Read the model definition and answer for the solid it produces. Units are mm, in the model's axes. Coordinates: 2 decimals unless noted, no trailing zeros. Loops run counter-clockwise (first coordinate to the right, second up) from the corner with the lowest first, then second, coordinate; pieces in that order, holes last. Notation, with made-up numbers: (-22, -38) - (-3, -38) arc R22 ccw to (-3, 0) - close; hole circle Ø8 at (62.25, 48.5). An arc over 180 degrees is marked (long way). One line per item, written item: value. Start each with the question number.
Autodesk Inventor part; units mm, degrees
ref_plane "Start plane" through (0, 0, 13.6102) normal (0, 0, 1) x (1, 0, 0)
ref_plane "End plane" through (0, 0, 536.3898) normal (0, 0, 1) x (1, 0, 0)
ref_plane "Work Plane4" through (0.6642, 2.6747, 533.4641) normal (-0.0396, -0.1596, 0.9864) x (0.9992, -0.0032, 0.0396)
ref_plane "Start plane" through (0, 0, 13.6102) normal (0, 0, 1) x (1, 0, 0)
ref_plane "End plane" through (0, 0, 536.3898) normal (0, 0, 1) x (1, 0, 0)
sketch "Sketch" plane through (0, 0, 0) normal (0, 0, 1) x (1, 0, 0)
  circle A0 centre (0, 0) radius 13.3858
  circle A1 centre (0, 0) radius 16.764
  dimension "d0" = 33.528
  dimension "d1" = 3.3782
extrude "Body" add sketch "Sketch" along normal up to surface (522.7796 mm away) from surface at 13.6102
sketch "Sketch3" plane through (0, 0, 0) normal (0, 0, 1) x (1, 0, 0)
  line L0 (0, 0) -> (10, 0)
ref_plane "Work Plane3" through (0, 0, 0) normal (0, -1, 0) x (1, 0, 0)
ref_plane "Work Plane4" through (0.6642, 2.6747, 533.4641) normal (-0.0396, -0.1596, 0.9864) x (0.9992, -0.0032, 0.0396)
split "Split1" plane through (0.6642, 2.6747, 533.4641) removes the side toward (-0.0396, -0.1596, 0.9864)
ref_plane "Work Plane5" through (0.6642, 2.6747, 16.5359) normal (-0.0396, -0.1596, -0.9864) x (0.8846, -0.4646, 0.0396)
split "Split2" plane through (0.6642, 2.6747, 16.5359) removes the side toward (-0.0396, -0.1596, -0.9864)
sketch "Sketch4" plane through (0, 0, 0) normal (0, -1, 0) x (1, 0, 0)
  line L0 (-2, 13.6102) -> (12, 13.6102)
  line L1 (-2, 536.3898) -> (12, 536.3898)
  dimension "d7" = 522.7796
equation "\"d0\" = G_H"
equation "\"d1\" = G_T"
equation "\"d2\" = G_L"
equation "\"G_H\" = 33.528"
equation "\"G_T\" = 3.3782"
equation "\"G_L\" = d7"
equation "\"G_OFFSET_START\" = -13.61022"
equation "\"G_OFFSET_END\" = -13.61022"
equation "\"d4\" = -G_OFFSET_START"
equation "\"d5\" = G_OFFSET_END + B_L"
equation "\"B_L\" = 550"
properties part number "ANSI - 1 x 0.133 - 20.582" material "Steel, Mild"
1) Determine the mould class of faces 1 (the flat face through (-11.254, 7.6, 16.217)), 2 (the cylindrical face through (15.486, 6.421, 271.348)), 3 (the cylindrical face through (12.365, 5.127, 271.356)) for opening direction X: released by +X, released by -X, zero draft, split by the parting line, or undercut.
2) Section C-C, the plane z = 221 is taken. Determine the outline of the cut face in (x, y).
3) Section B-B, the plane y = 6 is taken. Determine the outline of the cut face in (x, z), and give its area (3 significant figures).
4) Straight lines are drawn through the part: L1, parallel to Y at x = 0, z = 158; L2, parallel to Z at x = -6.5, y = 15. For each, find the intervals that lie inside material, in ascending order.
5) Section A-A, the plane x = -6 is taken. Determine the outline of the cut face in (y, z).
6) Flat-ended cylindrical pins translate along their axes: P1, Ø10, axis at y = -6.5, z = 479, coming from the -X side; P2, Ø3, axis at y = -3.5, z = 433.5, coming from the +X side; P3, Ø5, axis at y = -7, z = 352, coming from the -X side. Find the tip coordinate at first contact, or state that the pin passes through.
Answer below:
1. face 1: released by -X
1. face 2: split by the parting line
1. face 3: undercut
2. outline: circle Ø33.53 at (0, 0); hole circle Ø26.77 at (0, 0)
3. outline: (-15.65, 16.65) - (-11.97, 16.5) - (-11.97, 533.5) - (-15.65, 533.35) - close; (11.97, 15.54) - (15.65, 15.4) - (15.65, 534.6) - (11.97, 534.46) - close
3. area: 3,820 mm2
4. L1: -16.76 to -13.39, 13.39 to 16.76
4. L2: 14.83 to 535.17
5. outline: (-15.65, 19.77) - (-11.97, 19.17) - (-11.97, 530.83) - (-15.65, 530.23) - close; (11.97, 15.3) - (15.65, 14.7) - (15.65, 535.3) - (11.97, 534.7) - close
6. P1: x = -16.7
6. P2: x = 16.64
6. P3: x = -16.15
